Answer from the drawing. Dimensions are ordinates in mm from the lowest x, y and z of the part. A direction names the side the tool comes from. Round coordinates to 2 decimals unless told otherwise and drop trailing zeros. Write each loop counter-clockwise with the first axis right and the second up, starting at its lowest first coordinate (ties: lowest second). Pieces come first, ordered by that corner, then holes. Notation, with made-up numbers: (6.25, 62) - (22.25, 62) arc R35 cw to (22.25, 99) - close; hole circle Ø11 at (27, -18). An arc over 180 degrees is marked (long way). Answer in a Markdown table with one row per item.
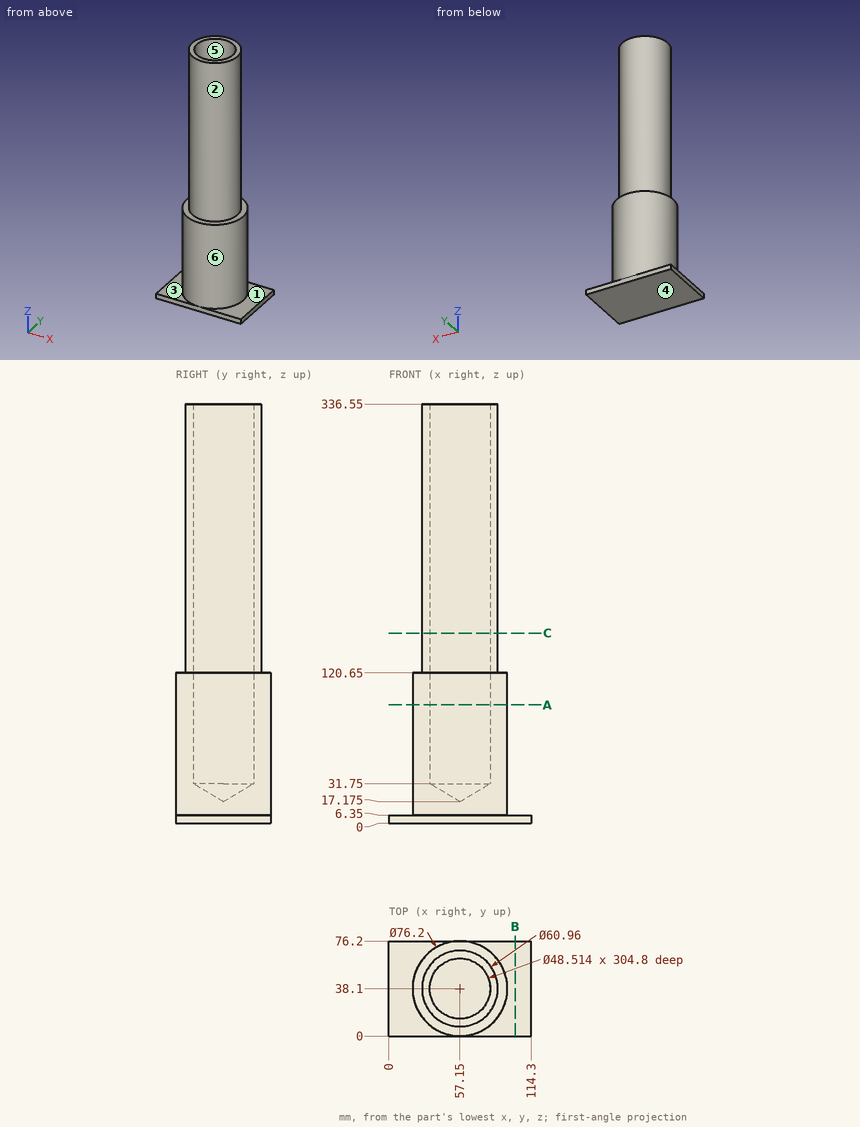
(1) Section C-C (z = 152.5) is taken. Give the vertices of the cut face in (x, y).
Checked values:
| item | result |
|---|---|
| outline | circle Ø60.96 at (57.15, 38.1); hole circle Ø48.51 at (57.15, 38.1) |
(2) Find the intervals of material crossed by line 1 (X direction, y = 38, z = 164); line 2 (Y direction, x = 57.15, z = 93.5); line 3 (Z direction, x = 83.5, y = 20), in increasing order.
Checked values:
| item | result |
|---|---|
| line 1 | x = 26.67 to 32.89, 81.41 to 87.63 |
| line 2 | y = 0 to 13.84, 62.36 to 76.2 |
| line 3 | z = 0 to 120.65 |
(3) Section B-B (x = 101.5) is taken. Give the vertices of the cut face in (y, z).
Checked values:
| item | result |
|---|---|
| outline | (0, 0) - (76.2, 0) - (76.2, 6.35) - (0, 6.35) - close |
(4) Flat-ended cylindrical pins translate along their axes: pin 1 (12 mm diameter, centred on x = 74.5, z = 178, fed in from -Y); pin 2 (1.5 mm diameter, centred on y = 58, z = 166, fed in from -X); pin 3 (1.5 mm diameter, centred on x = 29, y = 17.5, fed in from +Z); pin 4 (4 mm diameter, centred on x = 20.5, y = 8, fed in from -Z). Find the tip coordinate at first contact, or state that the pin passes through.
Checked values:
| item | result |
|---|---|
| pin 1 | stops at y = 9.81 |
| pin 2 | stops at x = 33.44 |
| pin 3 | stops at z = 120.65 |
| pin 4 | stops at z = 0 |
(5) For the marked faces 1, 2 and 3, determine the directions among +Z, -Z, +X, -X, +Y, -Y from which every point of the face is accessible in a straight line to the end or side of a thin tool.
Checked values:
| item | result |
|---|---|
| face 1 | +Z, +X |
| face 2 | +Z |
| face 3 | +Z, -X |
(6) For a pull along Y with two mould halves and no side action, classify the marked faces 4, 5 and 6 as pulls with the +Y half, pulls with the -Y half, needs draft (parallel to the pull), parting line crosses it, or undercut.
Checked values:
| item | result |
|---|---|
| face 4 | needs draft |
| face 5 | undercut |
| face 6 | parting line crosses it |
(7) Section A-A (z = 95) is taken. Give the vertices of the cut face in (x, y), and give its area (3 significant figures).
Checked values:
| item | result |
|---|---|
| outline | circle Ø76.2 at (57.15, 38.1); hole circle Ø48.51 at (57.15, 38.1) |
| area | 2,710 mm2 |
